```python
from build123d import *

# Parameters (mm, degrees)
SKETCH1_W           = 179.3875
SKETCH1_H           = 82.005714286
BOSS_EXTRUDE1_DEPTH = 163.5125
SKETCH2_W           = 46.0375
SKETCH2_H           = 25.4
CUT_EXTRUDE1_DEPTH  = 12.7
SKETCH3_R           = 6.380960286
BOSS_EXTRUDE2_DEPTH = 9.525


with BuildPart() as part:
    # Sketch1 → Boss-Extrude1 (new body)
    with BuildSketch(Plane(origin=(0, 0, 0), x_dir=(1, 0, 0), z_dir=(0, 1, 0))):
        with Locations((89.69375, 41.002857143)):
            Rectangle(SKETCH1_W, SKETCH1_H)
    extrude(amount=BOSS_EXTRUDE1_DEPTH)

    # Sketch2 → Cut-Extrude1 (cut)
    with BuildSketch(Plane(origin=(0, 163.5125, 0), x_dir=(1, 0, 0), z_dir=(0, 1, 0))):
        with Locations((23.01875, 12.7)):
            Rectangle(SKETCH2_W, SKETCH2_H)
        with Locations((156.36875, 12.7)):
            Rectangle(SKETCH2_W, SKETCH2_H)
    extrude(amount=-CUT_EXTRUDE1_DEPTH, mode=Mode.SUBTRACT)

    # Sketch3 → Boss-Extrude2 (add)
    with BuildSketch(Plane(origin=(0, 150.8125, 0), x_dir=(1, 0, 0), z_dir=(0, 1, 0))):
        with Locations((23.01875, 14.886216264)):
            Circle(SKETCH3_R)
        with Locations((156.36875, 14.886216264)):
            Circle(SKETCH3_R)
    extrude(amount=BOSS_EXTRUDE2_DEPTH)


solid = part.part
```
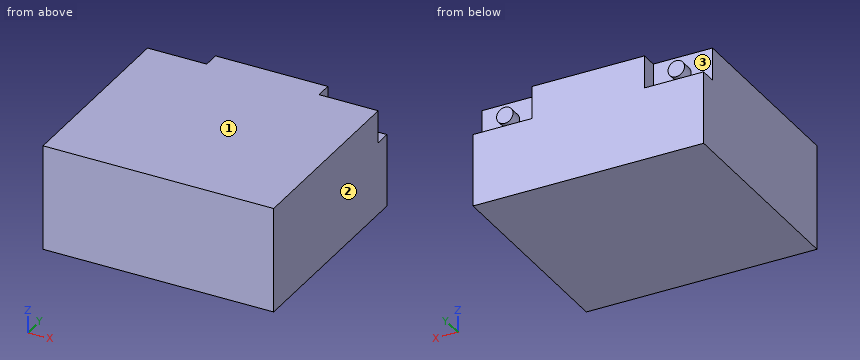
Can you work these out from the model? Positions are in its coordinate system, mm. Face numbers are marked on the shaded views. Coordinates: 2 decimals unless noted, no trailing zeros. Loops run counter-clockwise (first coordinate to the right, second up) from the corner with the lowest first, then second, coordinate; pieces in that order, holes last. Notation, with made-up numbers: M 7.5,-14.5 L 13.5,-14.5 A29 ccw 13.5,20.5 Z; hole C -6,12 d2. An arc over 180 degrees is marked long. Put each result on its own line as item: value. Start each with the question number.
(1) Imagine slicing it at C-C on x = 27. List the corners of the cut face in (y, z) for me.
(2) Imagine slicing it at B-B on z = -18.5. List the corners of the cut face in (x, y) for me, and give its area (3 significant figures).
(3) I need wall thicknesses on probe 1 along Y at (x, z) = (15.5, -12). Which ranges of the line are inside material? Lowest first, please.
(4) Will these pins go through, and if not, where does the flat tip stop? pin 1 Ø14 at (y, z) = (158, -10.5) entering from -X; pin 2 Ø4 at (x, y) = (145.5, 156) entering from +Z; pin 3 Ø7.5 at (x, z) = (30.5, -8.5) entering from +Y.
(5) Imagine slicing it at A-A on x = 147.5. List the corners of the cut face in (y, z) for me.
(6) We'd pull the mould along X, two halves only. Please class the marked faces 1, 2 and 3: +X half, -X half, draft (parallel to the pull), parting line (faces both ways), or undercut.
Worked answers:
1. outline: M 0,-82.01 L 163.51,-82.01 L 163.51,-25.4 L 150.81,-25.4 L 150.81,-19.87 L 160.34,-19.87 L 160.34,-9.9 L 150.81,-9.9 L 150.81,0 L 0,0 Z
2. outline: M 0,0 L 179.39,0 L 179.39,150.81 L 161.63,150.81 L 161.63,160.34 L 151.11,160.34 L 151.11,150.81 L 133.35,150.81 L 133.35,163.51 L 46.04,163.51 L 46.04,150.81 L 28.28,150.81 L 28.28,160.34 L 17.76,160.34 L 17.76,150.81 L 0,150.81 Z
2. area: 28,400 mm2
3. probe 1: y = 0 to 150.81
4. pin 1: stops at x = 16.64
4. pin 2: stops at z = -25.4
4. pin 3: stops at y = 160.34
5. outline: M 0,-82.01 L 163.51,-82.01 L 163.51,-25.4 L 150.81,-25.4 L 150.81,0 L 0,0 Z
6. face 1: draft
6. face 2: +X half
6. face 3: undercut
